Check sheet for the modelled part. Datum: model origin and axes. Units: mm. A direction names the side the tool comes from. Round coordinates to 2 decimals unless told otherwise and drop trailing zeros. Write each loop counter-clockwise with the first axis right and the second up, starting at its lowest first coordinate (ties: lowest second). Pieces come first, ordered by that corner, then holes. Notation, with made-up numbers: M 43,13.25 L 61,13.25 A16 cw 61,35.25 Z; hole C -20.75,1.5 d5. An arc over 180 degrees is marked long. Put each result on its own line as item: value.
```python
from build123d import *

# Parameters (mm, degrees)
SKETCH1_W           = 93.5
SKETCH1_H           = 123
BOSS_EXTRUDE1_DEPTH = 5
BOSS_EXTRUDE2_DEPTH = 30
CHAMFER1_SIZE       = 5
SKETCH4_W           = 6
SKETCH4_H           = 48.8
BOSS_EXTRUDE3_DEPTH = 14.6
SKETCH5_R           = 2.1
CUT_EXTRUDE1_DEPTH  = 3.5
SKETCH6_R           = 2.1
CUT_EXTRUDE2_DEPTH  = 3.5


with BuildPart() as part:
    # Sketch1 → Boss-Extrude1 (new body)
    with BuildSketch(Plane.XY):
        with Locations((0, 28.5)):
            Rectangle(SKETCH1_W, SKETCH1_H)
    extrude(amount=BOSS_EXTRUDE1_DEPTH)

    # Sketch3 → Boss-Extrude2 (add)
    with BuildSketch(Plane.XY.offset(5)):
        Polygon((-40.75, -22.4), (-46.75, -22.4), (-46.75, -33), (46.75, -33), (46.75, -22.4), (40.75, -22.4), (40.75, -27), (32.264718626, -27), (-32.264718626, -27), (-40.75, -27), align=None)
        Polygon((-36.864718626, -22.4), (-40.75, -22.4), (-40.75, -27), (-32.264718626, -27), align=None)
        Polygon((40.75, -27), (40.75, -22.4), (36.864718626, -22.4), (32.264718626, -27), align=None)
        Polygon((-46.75, 90), (-46.75, 26.4), (-40.75, 26.4), (-40.75, 75.514718626), (-40.75, 84), (-32.264718626, 84), (32.264718626, 84), (40.75, 84), (40.75, 75.514718626), (40.75, 26.4), (46.75, 26.4), (46.75, 90), align=None)
        Polygon((40.75, 84), (32.264718626, 84), (40.75, 75.514718626), align=None)
        Polygon((-40.75, 84), (-40.75, 75.514718626), (-32.264718626, 84), align=None)
    extrude(amount=BOSS_EXTRUDE2_DEPTH)

    # Chamfer1
    chamfer1_edges = [part.edges().sort_by_distance(p)[0] for p in [
        (-46.75, 90, 17.5),
        (46.75, 90, 17.5),
        (46.75, -33, 17.5),
        (-46.75, -33, 17.5),
    ]]
    chamfer(chamfer1_edges, length=CHAMFER1_SIZE)

    # Sketch4 → Boss-Extrude3 (add)
    with BuildSketch(Plane.XY.offset(5)):
        with Locations((-43.75, 2)):
            Rectangle(SKETCH4_W, SKETCH4_H)
    extrude(amount=BOSS_EXTRUDE3_DEPTH)

    # Sketch5 → Cut-Extrude1 (cut)
    with BuildSketch(Plane.XY.offset(35)):
        with Locations((-39.25, 82.5)):
            Circle(SKETCH5_R)
        with Locations(Location((-39.25, -25.5, 0), (0, 0, 180))):
            Circle(SKETCH5_R)
        with Locations(Location((39.25, 82.5, 0), (0, 0, 180))):
            Circle(SKETCH5_R)
        with Locations((39.25, -25.5)):
            Circle(SKETCH5_R)
    extrude(amount=-CUT_EXTRUDE1_DEPTH, mode=Mode.SUBTRACT)

    # Sketch6 → Cut-Extrude2 (cut)
    with BuildSketch(Plane(origin=(0, 0, 0), x_dir=(-1, 0, 0), z_dir=(0, 0, -1))):
        with Locations((-33.307444613, -24)):
            Circle(SKETCH6_R)
        with Locations((-33.307444613, 32)):
            Circle(SKETCH6_R)
        with Locations(Location((33.307444613, 32, 0), (0, 0, 180))):
            Circle(SKETCH6_R)
        with Locations(Location((33.307444613, -24, 0), (0, 0, 180))):
            Circle(SKETCH6_R)
    extrude(amount=-CUT_EXTRUDE2_DEPTH, mode=Mode.SUBTRACT)


solid = part.part
```
1. Cross-section at D-D (z = 17). Enter the section's corners in (x, y).
Computed values:
outline: M -46.75,-28 L -41.75,-33 L 41.75,-33 L 46.75,-28 L 46.75,-22.4 L 36.86,-22.4 L 32.26,-27 L -32.26,-27 L -36.86,-22.4 L -40.75,-22.4 L -40.75,75.51 L -32.26,84 L 32.26,84 L 40.75,75.51 L 40.75,26.4 L 46.75,26.4 L 46.75,85 L 41.75,90 L -41.75,90 L -46.75,85 Z
2. Cross-section at C-C (y = 32). Enter the section's corners in (x, z).
Computed values:
outline: M -46.75,0 L -35.41,0 L -35.41,3.5 L -31.21,3.5 L -31.21,0 L 31.21,0 L 31.21,3.5 L 35.41,3.5 L 35.41,0 L 46.75,0 L 46.75,35 L 40.75,35 L 40.75,5 L -40.75,5 L -40.75,35 L -46.75,35 Z
3. Release check for a two-part mould opening along X. For faces 1 (the flat face through (42, -22.4, 20)), 2 (the flat face through (-44.215, 87.535, 17.745)), 3 (the flat face through (-33, -24, 3.5)) record: +X half, -X half, draft (parallel to the pull), parting line (faces both ways), or undercut.
Computed values:
face 1: draft
face 2: -X half
face 3: undercut
4. Access from +Z, -Z, +X, -X, +Y, -Y to the whole of each face (thin tool, end or side, straight path). Record for faces 4 (the flat face through (-39, 83, 31.5)), 5 (the flat face through (-1, -33, 17)), 6 (the flat face through (33, -24, 3.5)).
Computed values:
face 4: +Z
face 5: +Z, -Z, +X, -X, -Y
face 6: -Z
5. Cross-section at A-A (z = 24). Enter the section's corners in (x, y), then the cut area to 3 significant figures.
Computed values:
outline: M -46.75,-28 L -41.75,-33 L 41.75,-33 L 46.75,-28 L 46.75,-22.4 L 36.86,-22.4 L 32.26,-27 L -32.26,-27 L -36.86,-22.4 L -46.75,-22.4 Z; M -46.75,26.4 L -40.75,26.4 L -40.75,75.51 L -32.26,84 L 32.26,84 L 40.75,75.51 L 40.75,26.4 L 46.75,26.4 L 46.75,85 L 41.75,90 L -41.75,90 L -46.75,85 Z
area: 1,950 mm2
6. Depth check by flat-ended pin: pin 1 Ø12 at (x, y) = (-3, 29.5) entering from +Z; pin 2 Ø5 at (x, y) = (-45, 6) entering from +Z; pin 3 Ø2 at (x, y) = (39, -26) entering from +Z. Enter the tip coordinate at first touch or a pass-through.
Computed values:
pin 1: stops at z = 5
pin 2: stops at z = 19.6
pin 3: stops at z = 31.5
7. Cross-section at B-B (x = 2). Enter the section's corners in (y, z).
Computed values:
outline: M -33,0 L 90,0 L 90,35 L 84,35 L 84,5 L -27,5 L -27,35 L -33,35 Z
8. Scan lines: probe 1 along Y at (x, z) = (19, 29); probe 2 along X at (y, z) = (55, 16); probe 3 along X at (y, z) = (82, 32). Record each from-to range of solid material in increasing order.
Computed values:
probe 1: y = -33 to -27, 84 to 90
probe 2: x = -46.75 to -40.75, 40.75 to 46.75
probe 3: x = -46.75 to -41.29, -37.21 to -34.26, 34.26 to 37.21, 41.29 to 46.75
